Read the model definition and answer for the solid it produces. Units are mm, in the model's axes. A direction names the side the tool comes from. Give positions to 0.01 mm unless a question says otherwise; leave off trailing zeros. Write each loop counter-clockwise with the first axis right and the second up, starting at its lowest first coordinate (ties: lowest second). Pieces come first, ordered by that corner, then holes. Notation, with made-up numbers: (42, 61.25) - (70, 61.25) arc R17 ccw to (70, 73.25) - close; hole circle Ø6 at (-26.5, 31). An arc over 180 degrees is marked (long way). Answer as CSV lines item,"result".
```python
from build123d import *
from OCP.BRepFilletAPI import BRepFilletAPI_MakeChamfer

# Parameters (mm, degrees)
ODGI_CIE_BAZOWE1_DEPTH     = 40
OTW_R_POD_RUB_M51_D        = 5.5
SZKIC4_R                   = 7
WYTNIJ_WYCI_GNI_CIE1_DEPTH = 69.85491994
OTW_R_POD_RUB_M61_D        = 6.6
SFAZOWANIE1_SIZE           = 4
SFAZOWANIE1_SIZE2          = 6.92820323


# Sheet-metal steps are written as plain solids
with BuildPart() as part:
    # Szkic1 → Odgięcie bazowe1 (new, symmetric)
    with BuildSketch(Plane.XY):
        with BuildLine():
            Line((-15, 54), (-15, 31))
            ThreePointArc((-15, 31), (-12.949747468, 26.050252532), (-8, 24))
            Line((-8, 24), (-4, 24))
            ThreePointArc((-4, 24), (-1.171572875, 22.828427125), (0, 20))
            Line((0, 20), (0, -20))
            ThreePointArc((0, -20), (-1.171572875, -22.828427125), (-4, -24))
            Line((-4, -24), (-8, -24))
            ThreePointArc((-8, -24), (-12.949747468, -26.050252532), (-15, -31))
            Line((-15, -31), (-15, -54))
            Line((-15, -54), (-12, -54))
            Line((-12, -54), (-12, -31))
            ThreePointArc((-12, -31), (-10.828427125, -28.171572875), (-8, -27))
            Line((-8, -27), (-4, -27))
            ThreePointArc((-4, -27), (0.949747468, -24.949747468), (3, -20))
            Line((3, -20), (3, 20))
            ThreePointArc((3, 20), (0.949747468, 24.949747468), (-4, 27))
            Line((-4, 27), (-8, 27))
            ThreePointArc((-8, 27), (-10.828427125, 28.171572875), (-12, 31))
            Line((-12, 31), (-12, 54))
            Line((-12, 54), (-15, 54))
        make_face()
    extrude(amount=ODGI_CIE_BAZOWE1_DEPTH, both=True)

    # Otwór pod śrubę M51 (through all)
    with Locations(Plane.ZY):
        with Locations((-14, 14), (14, 14), (14, -14), (-14, -14)):
            Hole(OTW_R_POD_RUB_M51_D / 2)

    # Szkic4 → Wytnij-wyciągnięcie1 (cut, through all)
    with BuildSketch(Plane.ZY):
        Circle(SZKIC4_R)
    extrude(amount=-WYTNIJ_WYCI_GNI_CIE1_DEPTH, mode=Mode.SUBTRACT)

    # Otwór pod śrubę M61 (through all)
    with Locations(Plane(origin=(-12, 0, 0), x_dir=(0, 0, -1), z_dir=(1, 0, 0))):
        with Locations((-32.50000905, 46.5), (-16.50000905, 46.5), (16.5, 46.5), (32.5, 46.5), (32.5, -46.5), (16.5, -46.5), (-16.49999095, -46.5), (-32.49999095, -46.5)):
            Hole(OTW_R_POD_RUB_M61_D / 2)

    # Sfazowanie1: one chamfer whose edges measure the first distance from different faces: ONE call of the kernel's chamfer builder (chamfer() names one face for all edges)
    sfazowanie1_edges_1 = [part.edges().sort_by_distance(p)[0] for p in [
        (-13.5, -54, -40),
        (-13.5, -54, 40),
    ]]
    sfazowanie1_side_1 = [part.faces().sort_by_distance(p)[0] for p in [
        (-13.5, -54, 0),
    ]]
    sfazowanie1_edges_2 = [part.edges().sort_by_distance(p)[0] for p in [
        (-13.5, 54, -40),
        (-13.5, 54, 40),
    ]]
    sfazowanie1_side_2 = [part.faces().sort_by_distance(p)[0] for p in [
        (-13.5, 54, 0),
    ]]
    sfazowanie1 = BRepFilletAPI_MakeChamfer(part.part.solid().wrapped)
    for e in sfazowanie1_edges_1:
        sfazowanie1.Add(SFAZOWANIE1_SIZE, SFAZOWANIE1_SIZE2, e.wrapped, sfazowanie1_side_1[0].wrapped)  # the first distance lies on this face
    for e in sfazowanie1_edges_2:
        sfazowanie1.Add(SFAZOWANIE1_SIZE, SFAZOWANIE1_SIZE2, e.wrapped, sfazowanie1_side_2[0].wrapped)  # the first distance lies on this face
    add(Compound.cast(sfazowanie1.Shape()), mode=Mode.REPLACE)


solid = part.part
```
(1) Find the intervals of material crossed by L1, parallel to Y at x = -13.4, z = -16.5; L2, parallel to Y at x = -13.8, z = -32.5; L3, parallel to Z at x = -13.5, y = 48.5, in increasing order.
Worked out:
L1,"y = -54 to -49.8, -43.2 to -26.55, 26.55 to 43.2, 49.8 to 54"
L2,"y = -54 to -49.8, -43.2 to -27.08, 27.08 to 43.2, 49.8 to 54"
L3,"z = -39.18 to -35.12, -29.88 to -19.12, -13.88 to 13.88, 19.12 to 29.88, 35.12 to 39.18"
(2) The mould has two halves that part along Z. Classify faces 6 (the cylindrical face through (-13.52, -43.23, -16.93)), 7 (the flat face through (1, 0, 40)), 8 (the cylindrical face through (-10.859, -28.203, 0.56)): +Z half, -Z half, draft (parallel to the pull), parting line (faces both ways), or undercut.
Worked out:
face 6,"undercut"
face 7,"+Z half"
face 8,"draft"
(3) A cutting plane is placed at D-D (y = 0). Write down the section's boundary in (x, z), and give its area (3 significant figures).
Worked out:
outline,"(0, -40) - (3, -40) - (3, -7) - (0, -7) - close; (0, 7) - (3, 7) - (3, 40) - (0, 40) - close"
area,"198 mm^2"
(4) A cutting plane is placed at A-A (y = 14). Write down the section's boundary in (x, z).
Worked out:
outline,"(0, -40) - (3, -40) - (3, -16.75) - (0, -16.75) - close; (0, -11.25) - (3, -11.25) - (3, 11.25) - (0, 11.25) - close; (0, 16.75) - (3, 16.75) - (3, 40) - (0, 40) - close"
(5) Each of these flat-tipped pins is pushed along its axis until it touches: P1, Ø3, axis at x = -2.5, y = -10.5, coming from the -Z side; P2, Ø3, axis at y = 28.5, z = 24.5, coming from the -X side; P3, Ø1, axis at y = 26, z = -4.5, coming from the -X side; P4, Ø18.5, axis at y = -47, z = -10, coming from the +X side. Where does it stop, or does it pass through?
Worked out:
P1,"passes through"
P2,"stops at x = -14.93"
P3,"stops at x = -13.36"
P4,"stops at x = -12"
(6) A cutting plane is placed at C-C (z = 0). Write down the section's boundary in (x, y), and give its area (3 significant figures).
Worked out:
outline,"(-15, -54) - (-12, -54) - (-12, -31) arc R4 cw to (-8, -27) - (-4, -27) arc R7 ccw to (3, -20) - (3, -7) - (0, -7) - (0, -20) arc R4 cw to (-4, -24) - (-8, -24) arc R7 ccw to (-15, -31) - close; (-15, 31) arc R7 ccw to (-8, 24) - (-4, 24) arc R4 cw to (0, 20) - (0, 7) - (3, 7) - (3, 20) arc R7 ccw to (-4, 27) - (-8, 27) arc R4 cw to (-12, 31) - (-12, 54) - (-15, 54) - close"
area,"344 mm^2"
(7) For faces 1 (the cylindrical face through (-13.52, 49.77, -16.93)), 2 (the flat face through (3, 9, 1)), 3 (the flat face through (-12, -43, 1)), 4 (the cylindrical face through (-13, 26.1, 0.6)), 5 (the flat face through (-12, 42, 1)), determine the directions among +Z, -Z, +X, -X, +Y, -Y from which every point of the face is accessible in a straight line to the end or side of a thin tool.
Worked out:
face 1,"+X, -X"
face 2,"+Z, -Z, +X, +Y, -Y"
face 3,"+Z, -Z, +X, -Y"
face 4,"+Z, -Z, -X"
face 5,"+Z, -Z, +X, +Y"
(8) A cutting plane is placed at B-B (x = -13.25). Count the separate pieces of the cut face and the enclosed holes in it, and give its area (3 significant figures).
Worked out:
separate pieces,"2"
enclosed holes,"8"
area,"4,090 mm^2"
